Work out the finished part from the listing and answer in its coordinate system (mm). A direction names the side the tool comes from. Coordinates: 2 decimals unless noted, no trailing zeros. Order: outer loops, then holes, each group sorted by start corner. A loop starts at its lowest first (then second) coordinate and runs counter-clockwise, first axis right, second up.
```python
from build123d import *

# Parameters (mm, degrees)
BOSS_EXTRUDE1_DEPTH = 75
SKETCH2_R           = 6.58
CUT_EXTRUDE1_DEPTH  = 15
SKETCH3_OUTSIDE_W   = 50.294
SKETCH3_OUTSIDE_H   = 46.118
SKETCH3_OUTSIDE_R   = 5.5
CUT_EXTRUDE3_DEPTH  = 2
SKETCH4_R           = 3.4
CUT_EXTRUDE4_DEPTH  = 76
SKETCH5_R           = 5.9
CUT_EXTRUDE5_DEPTH  = 36
SKETCH7_R           = 9.5
CUT_EXTRUDE7_DEPTH  = 19
SKETCH8_R           = 4.4
CUT_EXTRUDE8_DEPTH  = 28
SKETCH9_R           = 2.5
CUT_EXTRUDE9_DEPTH  = 34.75000005
CHAMFER2_SIZE       = 0.5
CHAMFER3_SIZE       = 2
CHAMFER4_SIZE       = 1


with BuildPart() as part:
    # Sketch1 → Boss-Extrude1 (new body)
    with BuildSketch(Plane(origin=(0, 0, 0), x_dir=(1, 0, 0), z_dir=(0, 1, 0))):
        Polygon((7.794228634, -13.5), (15.588457268, 0), (7.794228634, 13.5), (-7.794228634, 13.5), (-15.588457268, 0), (-7.794228634, -13.5), align=None)
    extrude(amount=BOSS_EXTRUDE1_DEPTH)

    # Sketch2 → Cut-Extrude1 (cut)
    with BuildSketch(Plane.XZ):
        Polygon((15.588457268, 0), (7.794228634, 13.5), (-7.794228634, 13.5), (-15.588457268, 0), (-7.794228634, -13.5), (7.794228634, -13.5), align=None)
        Circle(SKETCH2_R, mode=Mode.SUBTRACT)
    extrude(amount=-CUT_EXTRUDE1_DEPTH, mode=Mode.SUBTRACT)

    # Sketch3 outside → Cut-Extrude3 (cut)
    with BuildSketch(Plane.XZ.offset(-15)):
        Rectangle(SKETCH3_OUTSIDE_W, SKETCH3_OUTSIDE_H)
        Circle(SKETCH3_OUTSIDE_R, mode=Mode.SUBTRACT)
    extrude(amount=-CUT_EXTRUDE3_DEPTH, mode=Mode.SUBTRACT)

    # Sketch4 → Cut-Extrude4 (cut, through all)
    with BuildSketch(Plane.XZ):
        Circle(SKETCH4_R)
    extrude(amount=-CUT_EXTRUDE4_DEPTH, mode=Mode.SUBTRACT)

    # Sketch5 → Cut-Extrude5 (cut)
    with BuildSketch(Plane(origin=(0, 75, 0), x_dir=(1, 0, 0), z_dir=(0, 1, 0))):
        Circle(SKETCH5_R)
    extrude(amount=-CUT_EXTRUDE5_DEPTH, mode=Mode.SUBTRACT)

    # Sketch7 → Cut-Extrude7 (cut)
    with BuildSketch(Plane(origin=(0, 75, 0), x_dir=(1, 0, 0), z_dir=(0, 1, 0))):
        Circle(SKETCH7_R)
    extrude(amount=-CUT_EXTRUDE7_DEPTH, mode=Mode.SUBTRACT)

    # Sketch8 → Cut-Extrude8 (cut, through all)
    with BuildSketch(Plane.XY.offset(13.5)):
        with Locations((0, 33)):
            Circle(SKETCH8_R)
    extrude(amount=-CUT_EXTRUDE8_DEPTH, mode=Mode.SUBTRACT)

    # Sketch9 → Cut-Extrude9 (cut, through all)
    with BuildSketch(Plane(origin=(-11.691342951, 0, -6.75), x_dir=(-0.5, 0, 0.866025404), z_dir=(-0.866025404, 0, -0.5))):
        with Locations((0, 33)):
            Circle(SKETCH9_R)
    extrude(amount=-CUT_EXTRUDE9_DEPTH, mode=Mode.SUBTRACT)

    # Sketch10 → Cut-Revolve1 (revolve, cut)
    with BuildSketch(Plane(origin=(0, 0, 0), x_dir=(0, 0, -1), z_dir=(1, 0, 0))):
        Polygon((8.51850403, 79.98149597), (18.48149597, 70.01850403), (18.48149597, 79.98149597), align=None)
        Polygon((16.279129623, 19.779129623), (10.720870377, 14.220870377), (16.279129623, 14.220870377), align=None)
    revolve(axis=Axis((0, 77.98149597, 0), (0, -1, 0)), mode=Mode.SUBTRACT)

    # Chamfer2
    chamfer2_edges = [part.edges().sort_by_distance(p)[0] for p in [
        (-10.441342951, 33, -8.915063509),
        (-3.4, 0, 0),
        (-3.4, 39, 0),
        (-5.9, 56, 0),
        (-4.4, 33, -13.5),
        (-4.4, 33, 13.5),
        (12.941342951, 33, 4.584936491),
    ]]
    chamfer(chamfer2_edges, length=CHAMFER2_SIZE)

    # Chamfer3
    chamfer3_edges = [part.edges().sort_by_distance(p)[0] for p in [
        (-9.5, 75, 0),
    ]]
    chamfer(chamfer3_edges, length=CHAMFER3_SIZE)

    # Chamfer4
    chamfer4_edges = [part.edges().sort_by_distance(p)[0] for p in [
        (-6.58, 0, 0),
        (-6.58, 15, 0),
    ]]
    chamfer(chamfer4_edges, length=CHAMFER4_SIZE)


solid = part.part
```
1. For faces 1 (the cylindrical face through (-1.426, 7.409, -6.424)), 2 (the conical face through (6.97, 17.5, -12.14)), 3 (the flat face through (1, 39, 4)), 4 (the flat face through (11.746, 45.594, -6.656)), 5 (the cylindrical face through (-1.19, 15.99, -5.37)), determine the directions among +Z, -Z, +X, -X, +Y, -Y from which every point of the face is accessible in a straight line to the end or side of a thin tool.
2. The part is cut by section C-C (y = 53.5). Determine the outline of the cut face in (x, z), plus the area to 3 significant figures.
3. The mould has two halves that part along X. Classify faces 6 (the flat face through (10, 75, -6)), 7 (the cylindrical face through (8.39, 33.11, 1.96)), 8 (the conical face through (14, 17.5, 0)), 9 (the conical face through (-14, 17.5, 0)): released by +X, released by -X, zero draft, split by the parting line, or undercut.
4. The part is cut by section D-D (y = 9.5). Determine the outline of the cut face in (x, z), plus the area to 3 significant figures.
5. Flat-ended cylindrical pins translate along their axes: pin 1 (6 mm diameter, centred on x = 0, z = 0, fed in from -Y); pin 2 (13.5 mm diameter, centred on x = 0, z = 0, fed in from +Y); pin 3 (4 mm diameter, centred on x = 3, z = -0.5, fed in from -Y); pin 4 (3.5 mm diameter, centred on x = -2, z = 1.5, fed in from +Y). Find the tip coordinate at first contact, or state that the pin passes through.
6. Consider probe 1 along Y at (x, z) = (-10, -5.75); probe 2 along Z at (x, y) = (0, 48.5); probe 3 along X at (y, z) = (46.5, 0). Determine where each line is inside the solid, lowest interval first.
7. The part is cut by section A-A (y = 23). Determine the outline of the cut face in (x, z).
8. The part is cut by section B-B (y = 33). Count the separate pieces of the cut face and the enclosed holes in it, plus the area to 3 significant figures.
Worked out:
1. face 1: -Y
1. face 2: -Z, +X, -Y
1. face 3: +Y
1. face 4: -Z, +X, +Y, -Y
1. face 5: none
2. outline: (-15.59, 0) - (-7.79, -13.5) - (7.79, -13.5) - (15.59, 0) - (7.79, 13.5) - (-7.79, 13.5) - close; hole circle Ø11.8 at (0, 0)
2. area: 522 mm2
3. face 6: zero draft
3. face 7: undercut
3. face 8: released by +X
3. face 9: released by -X
4. outline: circle Ø13.16 at (0, 0); hole circle Ø6.8 at (0, 0)
4. area: 99.7 mm2
5. pin 1: passes through
5. pin 2: stops at y = 56
5. pin 3: stops at y = 0
5. pin 4: stops at y = 39
6. probe 1: y = 17 to 30.5, 35.5 to 75
6. probe 2: z = -13.5 to -5.9, 5.9 to 13.5
6. probe 3: x = -15.59 to -5.9, 5.9 to 15.59
7. outline: (-15.59, 0) - (-7.79, -13.5) - (7.79, -13.5) - (15.59, 0) - (7.79, 13.5) - (-7.79, 13.5) - close; hole circle Ø6.8 at (0, 0)
8. separate pieces: 4
8. enclosed holes: 0
8. area: 309 mm2
